Verification items for the finished model (mm, model axes). A direction names the side the tool comes from. Round coordinates to 2 decimals unless told otherwise and drop trailing zeros. Write each loop counter-clockwise with the first axis right and the second up, starting at its lowest first coordinate (ties: lowest second). Pieces come first, ordered by that corner, then holes. Notation, with made-up numbers: M 35.5,0 L 44.5,0 A22 cw 44.5,10 Z; hole C -23,79.5 d5. An arc over 180 degrees is marked long. Answer in a Markdown table with one row per item. Add a question column.
1. Sectioned sample at C-C on x = -35. Record the cut outline in (y, z).
2. Draft check along X on faces 3 (the flat face through (24, 12.4, -23)), 4 (the flat face through (8, -10, 13)), 5 (the cylindrical face through (-39.05, 14.93, -8.67)). Enter one of: pulls with the +X half, pulls with the -X half, needs draft (parallel to the pull), parting line crosses it, or undercut.
3. Go/stop test with flat-tipped pins: pin 1 Ø6 at (x, y) = (-30, 3.5) entering from +Z; pin 2 Ø1.5 at (x, y) = (22.5, 0.5) entering from -Z; pin 3 Ø4 at (x, z) = (0, 35) entering from -Y. Record where each tip stops, or that it passes through.
4. Sectioned sample at D-D on y = 2.25. Record the cut outline in (x, z), plus the area to 3 significant figures.
5. Sectioned sample at A-A on x = 0. Record the cut outline in (y, z).
6. Material ranges on probe 1 along X at (y, z) = (10.5, -23); probe 2 along Z at (x, y) = (-22.5, 10.5); probe 3 along Z at (x, y) = (25.5, 13.25), recorded low to high.
7. Set-up check for faces 1 (the cylindrical face through (21.252, 11.183, 24.595)), 2 (the cylindrical face through (-23.964, 16.147, 26.257)): record each of +Z, -Z, +X, -X, +Y, -Y from which the full face is reachable in a straight line by a thin tool's end or side.
8. Sectioned sample at B-B on z = 11. Record the cut outline in (x, y).
```python
from build123d import *

# Parameters (mm, degrees)
CROQUIS1_R                                     = 15
SALIENTE_EXTRUIR1_DEPTH                        = 10
CROQUIS2_R                                     = 40
CROQUIS2_R_2                                   = 15
SALIENTE_EXTRUIR2_DEPTH                        = 10
REFRENTADO_START                               = 10
REFRENTADO_PARA_TORNILLO_CON_CABEZA_2_R        = 3.5
REFRENTADO_PARA_TORNILLO_CON_CABEZA_TRON_DEPTH = 2.4
REFRENTADO_START_2                             = 12.4
REFRENTADO_PARA_TORNILLO_CON_CABEZA_3_OU_R     = 1.7
REFRENTADO_PARA_TORNILLO_CON_CABEZA_3_DEPTH    = 7.6


# Read off the part's stored shape, not the designer's step: Refrentado para tornillo con cabeza troncocónica de M31
with BuildPart() as part:
    # Croquis1 → Saliente-Extruir1 (new, symmetric)
    with BuildSketch(Plane(origin=(0, 0, 0), x_dir=(1, 0, 0), z_dir=(0, 1, 0))):
        with BuildLine():
            ThreePointArc((29.895833333, 2.497828918), (-30, 0), (29.895833333, -2.497828918))
            ThreePointArc((29.895833333, -2.497828918), (32.5, 0), (29.895833333, 2.497828918))
        make_face()
        with Locations(Location((0, 0, 0), (0, 0, 270))):
            Circle(CROQUIS1_R, mode=Mode.SUBTRACT)
    extrude(amount=SALIENTE_EXTRUIR1_DEPTH, both=True)

    # Croquis2 → Saliente-Extruir2 (add)
    with BuildSketch(Plane(origin=(0, 10, 0), x_dir=(1, 0, 0), z_dir=(0, 1, 0))):
        with Locations(Location((0, 0, 0), (0, 0, 270))):
            Circle(CROQUIS2_R)
        with Locations(Location((0, 0, 0), (0, 0, 270))):
            Circle(CROQUIS2_R_2, mode=Mode.SUBTRACT)
    extrude(amount=SALIENTE_EXTRUIR2_DEPTH)

    # Refrentado para tornillo con cabeza  2 → Refrentado para tornillo con cabeza troncocónica de M31 (cut)
    with BuildSketch(Plane(origin=(0, 0, 0), x_dir=(1, 0, 0), z_dir=(0, 1, 0)).offset(REFRENTADO_START)):
        with Locations((-24.748737342, -24.748737342)):
            Circle(REFRENTADO_PARA_TORNILLO_CON_CABEZA_2_R)
        with Locations((-35, 0)):
            Circle(REFRENTADO_PARA_TORNILLO_CON_CABEZA_2_R)
        with Locations((-24.748737342, 24.748737342)):
            Circle(REFRENTADO_PARA_TORNILLO_CON_CABEZA_2_R)
        with Locations((0, 35)):
            Circle(REFRENTADO_PARA_TORNILLO_CON_CABEZA_2_R)
        with Locations((24.748737342, 24.748737342)):
            Circle(REFRENTADO_PARA_TORNILLO_CON_CABEZA_2_R)
        with Locations((35, 0)):
            Circle(REFRENTADO_PARA_TORNILLO_CON_CABEZA_2_R)
        with Locations((24.748737342, -24.748737342)):
            Circle(REFRENTADO_PARA_TORNILLO_CON_CABEZA_2_R)
        with Locations((0, -35)):
            Circle(REFRENTADO_PARA_TORNILLO_CON_CABEZA_2_R)
    extrude(amount=REFRENTADO_PARA_TORNILLO_CON_CABEZA_TRON_DEPTH, mode=Mode.SUBTRACT)

    # Refrentado para tornillo con cabeza 3 ou → Refrentado para tornillo con cabeza  3 (cut)
    with BuildSketch(Plane(origin=(0, 0, 0), x_dir=(1, 0, 0), z_dir=(0, 1, 0)).offset(REFRENTADO_START_2)):
        with Locations((-24.748737342, -24.748737342)):
            Circle(REFRENTADO_PARA_TORNILLO_CON_CABEZA_3_OU_R)
        with Locations((-35, 0)):
            Circle(REFRENTADO_PARA_TORNILLO_CON_CABEZA_3_OU_R)
        with Locations((-24.748737342, 24.748737342)):
            Circle(REFRENTADO_PARA_TORNILLO_CON_CABEZA_3_OU_R)
        with Locations((0, 35)):
            Circle(REFRENTADO_PARA_TORNILLO_CON_CABEZA_3_OU_R)
        with Locations((24.748737342, 24.748737342)):
            Circle(REFRENTADO_PARA_TORNILLO_CON_CABEZA_3_OU_R)
        with Locations((35, 0)):
            Circle(REFRENTADO_PARA_TORNILLO_CON_CABEZA_3_OU_R)
        with Locations((24.748737342, -24.748737342)):
            Circle(REFRENTADO_PARA_TORNILLO_CON_CABEZA_3_OU_R)
        with Locations((0, -35)):
            Circle(REFRENTADO_PARA_TORNILLO_CON_CABEZA_3_OU_R)
    extrude(amount=REFRENTADO_PARA_TORNILLO_CON_CABEZA_3_DEPTH, mode=Mode.SUBTRACT)


solid = part.part
```
Geometry check:
| question | item | result |
|---|---|---|
| 1 | outline | M 10,-19.36 L 20,-19.36 L 20,-1.7 L 12.4,-1.7 L 12.4,-3.5 L 10,-3.5 Z; M 10,3.5 L 12.4,3.5 L 12.4,1.7 L 20,1.7 L 20,19.36 L 10,19.36 Z |
| 2 | face 3 | undercut |
| 2 | face 4 | needs draft |
| 2 | face 5 | parting line crosses it |
| 3 | pin 1 | stops at z = 13.08 |
| 3 | pin 2 | stops at z = -20.66 |
| 3 | pin 3 | stops at y = 12.4 |
| 4 | outline | M 29.9,-2.5 A2.5 ccw long 29.9,2.5 A30 ccw long Z; hole C 0,0 d30 |
| 4 | area | 2,130 mm2 |
| 5 | outline | M -10,-30 L 10,-30 L 10,-31.5 L 12.4,-31.5 L 12.4,-33.3 L 20,-33.3 L 20,-15 L -10,-15 Z; M -10,15 L 20,15 L 20,33.3 L 12.4,33.3 L 12.4,31.5 L 10,31.5 L 10,30 L -10,30 Z; M 10,-40 L 20,-40 L 20,-36.7 L 12.4,-36.7 L 12.4,-38.5 L 10,-38.5 Z; M 10,38.5 L 12.4,38.5 L 12.4,36.7 L 20,36.7 L 20,40 L 10,40 Z |
| 6 | probe 1 | x = -32.73 to -27.78, -21.72 to 21.72, 27.78 to 32.73 |
| 6 | probe 2 | z = -33.07 to -27.43, -22.07 to 22.07, 27.43 to 33.07 |
| 6 | probe 3 | z = -30.82 to -26.27, -23.22 to 23.22, 26.27 to 30.82 |
| 7 | face 1 | -Y |
| 7 | face 2 | +Y, -Y |
| 8 | outline | M -38.46,10 L -27.91,10 L -27.91,-10 L -10.2,-10 L -10.2,20 L -38.46,20 Z; M 10.2,-10 L 27.91,-10 L 27.91,10 L 38.46,10 L 38.46,20 L 10.2,20 Z |
